from build123d import *

# Parameters (mm, degrees)
SKETCH1_W                        = 25.4
SKETCH1_H                        = 25.4
BOSS_EXTRUDE1_DEPTH              = 89.408
F_3_8_0_375_DIAMETER_HOLE1_D     = 9.525
F_3_8_0_375_DIAMETER_HOLE1_DEPTH = 25.4
F_3_8_0_375_DIAMETER_HOLE1_TIP   = 2.861598698
F_3_8_0_375_DIAMETER_HOLE2_D     = 9.525
F_3_8_0_375_DIAMETER_HOLE2_DEPTH = 25.4
F_3_8_0_375_DIAMETER_HOLE2_TIP   = 2.861598698


with BuildPart() as part:
    # Sketch1 → Boss-Extrude1 (new body)
    with BuildSketch(Plane.XY):
        with Locations((12.7, 12.7)):
            Rectangle(SKETCH1_W, SKETCH1_H)
    extrude(amount=BOSS_EXTRUDE1_DEPTH)

    # 3/8 (0.375) Diameter Hole1
    with Locations(Plane(origin=(0, 0, 0), x_dir=(-1, 0, 0), z_dir=(0, 0, -1))):
        with Locations((-12.7, 12.7)):
            Hole(F_3_8_0_375_DIAMETER_HOLE1_D / 2, depth=F_3_8_0_375_DIAMETER_HOLE1_DEPTH)
            with Locations((0, 0, -(F_3_8_0_375_DIAMETER_HOLE1_DEPTH + F_3_8_0_375_DIAMETER_HOLE1_TIP / 2))):  # 118° drill point
                Cone(0, F_3_8_0_375_DIAMETER_HOLE1_D / 2, F_3_8_0_375_DIAMETER_HOLE1_TIP, mode=Mode.SUBTRACT)

    # 3/8 (0.375) Diameter Hole2
    with Locations(Plane.XY.offset(89.408)):
        with Locations((12.7, 12.7)):
            Hole(F_3_8_0_375_DIAMETER_HOLE2_D / 2, depth=F_3_8_0_375_DIAMETER_HOLE2_DEPTH)
            with Locations((0, 0, -(F_3_8_0_375_DIAMETER_HOLE2_DEPTH + F_3_8_0_375_DIAMETER_HOLE2_TIP / 2))):  # 118° drill point
                Cone(0, F_3_8_0_375_DIAMETER_HOLE2_D / 2, F_3_8_0_375_DIAMETER_HOLE2_TIP, mode=Mode.SUBTRACT)


solid = part.part
Part model, mm, in its own coordinate system. A direction names the side the tool comes from. Coordinates: 2 decimals unless noted, no trailing zeros. Order: outer loops, then holes, each group sorted by start corner. A loop starts at its lowest first (then second) coordinate and runs counter-clockwise, first axis right, second up.
(1) Probe L1, parallel to X at y = 12.7, z = 19; L2, parallel to Y at x = 14.25, z = 10.5. List the from-to ranges inside material, lowest first.
Check sheet entries:
L1: x = 0 to 7.94, 17.46 to 25.4
L2: y = 0 to 8.2, 17.2 to 25.4
(2) Tool access for faces 1 (the face through (13.73, 8.05, 76.53)), 2 (the face through (7.942, 12.909, 12.878)), 3 (the face through (18, 13, 0)): list every direction of +Z, -Z, +X, -X, +Y, -Y with a clear straight run to the whole face (end or side of a thin tool).
Check sheet entries:
face 1: +Z
face 2: -Z
face 3: -Z, +X, -X, +Y, -Y
(3) Pull direction Y, two halves, no side cores. Call faces 4 (the face through (13, 0, 44)), 5 (the face through (12.044, 12.197, 61.643)), 6 (the face through (13, 25.4, 44)), 7 (the face through (0, 13, 44)): pulls with the +Y half, pulls with the -Y half, needs draft (parallel to the pull), parting line crosses it, or undercut.
Check sheet entries:
face 4: pulls with the -Y half
face 5: undercut
face 6: pulls with the +Y half
face 7: needs draft
(4) Slice it at A-A, the plane z = 17. Write the cut outline in (x, y) (1 decimal), and give its area (3 significant figures).
Check sheet entries:
outline: (0, 0) - (25.4, 0) - (25.4, 25.4) - (0, 25.4) - close; hole circle Ø9.5 at (12.7, 12.7)
area: 574 mm2
